Design review of the part built by this model. Coordinates are the model's own, in mm. Give positions to 0.01 mm unless a question says otherwise; leave off trailing zeros. Loops run counter-clockwise (first coordinate to the right, second up) from the corner with the lowest first, then second, coordinate; pieces in that order, holes last. Notation, with made-up numbers: M 2,70 L 24,70 A4 cw 24,77 Z; hole C -7.75,33 d6. An arc over 180 degrees is marked long. Answer as CSV lines item,"result".
```python
from build123d import *

# Parameters (mm, degrees)
SKETCH1_W              = 146.05
SKETCH1_H              = 101.6
BOSS_EXTRUDE2_DEPTH    = 4.7625
SKETCH2_R              = 11.1125
SKETCH2_R_2            = 14.2875
CUT_EXTRUDE1_DEPTH     = 5.7625
F_10_CLEARANCE_HOLE1_D = 5.1054
F_10_CLEARANCE_HOLE2_D = 5.6134
CUT_EXTRUDE2_DEPTH     = 5.7625
FILLET1_R              = 4.7625
SKETCH8_R              = 14.2875
CUT_EXTRUDE3_DEPTH     = 5.7625001
SKETCH9_R              = 14.2875
SKETCH9_R_2            = 11.1125
BOSS_EXTRUDE3_DEPTH    = 4.7625


with BuildPart() as part:
    # Sketch1 → Boss-Extrude2 (new body)
    with BuildSketch(Plane(origin=(0, 0, 0), x_dir=(0, 0, -1), z_dir=(1, 0, 0))):
        with Locations((73.025, 50.8)):
            Rectangle(SKETCH1_W, SKETCH1_H)
    extrude(amount=BOSS_EXTRUDE2_DEPTH)

    # Sketch2 → Cut-Extrude1 (cut, through all)
    with BuildSketch(Plane(origin=(4.7625, 0, 0), x_dir=(0, 0, -1), z_dir=(1, 0, 0))):
        with Locations((66.2432, 57.15)):
            Circle(SKETCH2_R)
        with Locations((31.75, 57.15)):
            Circle(SKETCH2_R)
        with Locations((90.633575625, 32.759624375)):
            Circle(SKETCH2_R_2)
    extrude(amount=-CUT_EXTRUDE1_DEPTH, mode=Mode.SUBTRACT)

    # #10 Clearance Hole1 (through all)
    with Locations(Plane(origin=(4.7625, 0, 0), x_dir=(0, 0, -1), z_dir=(1, 0, 0))):
        with Locations((9.525, 84.829624375), (111.125, 61.334624375), (9.525, 32.759624375), (111.125, 16.884624375)):
            Hole(F_10_CLEARANCE_HOLE1_D / 2)

    # #10 Clearance Hole2 (through all)
    with Locations(Plane(origin=(4.7625, 0, 0), x_dir=(0, 0, -1), z_dir=(1, 0, 0))):
        with Locations((9.525, 58.794624375), (48.9966, 84.829624375), (125.056959494, 58.794624375), (63.5, 32.759624375)):
            Hole(F_10_CLEARANCE_HOLE2_D / 2)

    # Sketch7 → Cut-Extrude2 (cut, through all)
    with BuildSketch(Plane(origin=(4.7625, 0, 0), x_dir=(0, 0, -1), z_dir=(1, 0, 0))):
        with BuildLine():
            ThreePointArc((58.52011675, 84.661535946), (82.426770011, 80.700428589), (94.694801926, 59.802729323))
            Line((94.694801926, 59.802729323), (104.928643901, 68.568627146))
            ThreePointArc((104.928643901, 68.568627146), (108.639710016, 70.529675147), (112.8333867, 70.705165442))
            Line((112.8333867, 70.705165442), (126.765346195, 68.165165442))
            ThreePointArc((126.765346195, 68.165165442), (133.252161891, 63.648929957), (134.095626133, 55.789939634))
            Line((134.095626133, 55.789939634), (120.163666639, 13.879939634))
            ThreePointArc((120.163666639, 13.879939634), (111.198276093, 7.359906237), (102.133632107, 13.741229966))
            ThreePointArc((102.133632107, 13.741229966), (93.170530223, 10.67989416), (83.746678665, 11.628574348))
            Line((83.746678665, 11.628574348), (31.75, 28.575))
            ThreePointArc((31.75, 28.575), (25.188529488, 29.338532406), (18.97770782, 31.588326004))
            ThreePointArc((18.97770782, 31.588326004), (8.938236412, 23.252714599), (0, 32.759624375))
            Line((0, 32.759624375), (0, 0))
            Line((0, 0), (146.05, 0))
            Line((146.05, 0), (146.05, 101.6))
            Line((146.05, 101.6), (0, 101.6))
            Line((0, 101.6), (0, 84.829624375))
            ThreePointArc((0, 84.829624375), (10.639110316, 94.28924293), (18.789371801, 82.616698681))
            ThreePointArc((18.789371801, 82.616698681), (28.938717529, 85.586373114), (39.47308325, 84.661535946))
            ThreePointArc((39.47308325, 84.661535946), (48.9966, 94.354624375), (58.52011675, 84.661535946))
        make_face()
    extrude(amount=-CUT_EXTRUDE2_DEPTH, mode=Mode.SUBTRACT)

    # Fillet1
    fillet1_edges = [part.edges().sort_by_distance(p)[0] for p in [
        (2.38125, 59.802729323, -94.694801926),
        (2.38125, 84.661535946, -58.52011675),
        (2.38125, 84.661535946, -39.47308325),
        (2.38125, 82.616698681, -18.789371801),
        (2.38125, 31.588326004, -18.97770782),
        (2.38125, 28.575, -31.75),
        (2.38125, 13.741229966, -102.133632107),
    ]]
    fillet(fillet1_edges, radius=FILLET1_R)

    # Sketch8 → Cut-Extrude3 (cut, through all)
    with BuildSketch(Plane(origin=(4.7625, 0, 0), x_dir=(0, 0, -1), z_dir=(1, 0, 0))):
        with Locations((31.75, 57.15)):
            Circle(SKETCH8_R)
    extrude(amount=-CUT_EXTRUDE3_DEPTH, mode=Mode.SUBTRACT)

    # Sketch9 → Boss-Extrude3 (add)
    with BuildSketch(Plane(origin=(4.7625, 0, 0), x_dir=(0, 0, -1), z_dir=(1, 0, 0))):
        with Locations((90.633575625, 32.759624375)):
            Circle(SKETCH9_R)
        with Locations((90.633575625, 32.759624375)):
            Circle(SKETCH9_R_2, mode=Mode.SUBTRACT)
    extrude(amount=-BOSS_EXTRUDE3_DEPTH)


solid = part.part
```
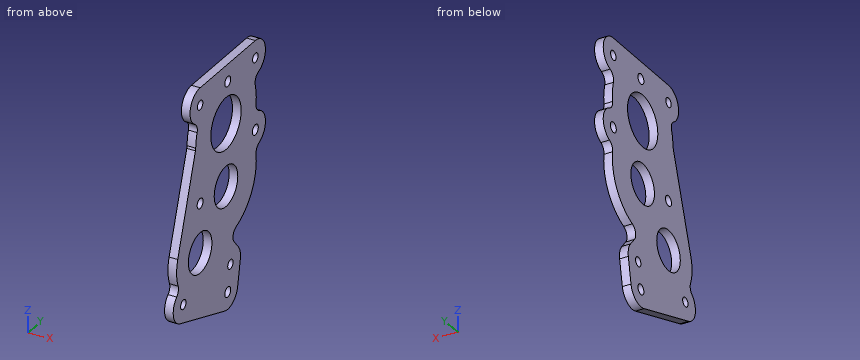
1. We need section A-A, the plane y = 47.5. Write out the cut boundary in (x, z), plus the area to 3 significant figures.
Answer block:
outline,"M 0,-131.34 L 4.76,-131.34 L 4.76,-71.75 L 0,-71.75 Z; M 0,-60.73 L 4.76,-60.73 L 4.76,-42.29 L 0,-42.29 Z; M 0,-21.21 L 4.76,-21.21 L 4.76,0 L 0,0 Z"
area,"473 mm²"
2. We need section D-D, the plane x = 1.8. Count the separate pieces of the cut face and the enclosed holes in it, plus the area to 3 significant figures.
Answer block:
separate pieces,"1"
enclosed holes,"11"
area,"6,520 mm²"
3. For P1, Ø1, axis at x = 3.5, z = -75, coming from the +Y side; P2, Ø17, axis at y = 57.15, z = -31.75, coming from the -X side; P3, Ø2, axis at x = 1.5, z = -86, coming from the -Y side; P4, Ø1.5, axis at x = 2, z = -27, coming from the -Y side, all flat-tipped, find the tip position at first contact; note any pin that passes through.
Answer block:
P1,"y = 84.51"
P2,"through"
P3,"y = 10.83"
P4,"y = 28.86"
4. We need section B-B, the plane z = -125. Write out the cut boundary in (x, y).
Answer block:
outline,"M 0,28.43 L 4.76,28.43 L 4.76,55.99 L 0,55.99 Z; M 0,61.6 L 4.76,61.6 L 4.76,68.49 L 0,68.49 Z"
5. We need section C-C, the plane z = -110.5. Write out the cut boundary in (x, y).
Answer block:
outline,"M 0,7.38 L 4.76,7.38 L 4.76,14.41 L 0,14.41 Z; M 0,19.36 L 4.76,19.36 L 4.76,58.86 L 0,58.86 Z; M 0,63.81 L 4.76,63.81 L 4.76,70.84 L 0,70.84 Z"
6. To check wall thickness, follow L1, parallel to Y at x = 2.15, z = -91; L2, parallel to Y at x = 0.45, z = -11; L3, parallel to Z at x = 1.45, y = 58. State the ranges of each line that lie inside material, in increasing order. Write a range as [from, to].
Answer block:
L1,"[10.54, 21.65], [43.87, 71.42]"
L2,"[23.35, 30.68], [34.84, 56.41], [61.18, 82.75], [86.91, 94.24]"
L3,"[-134.55, -127.75], [-122.37, -77.32], [-55.16, -46.01], [-17.49, -12.22], [-6.83, 0]"
